Check sheet for the drawn part. Datum: minimum x, y, z corner. Units: mm. Round coordinates to 2 decimals unless told otherwise and drop trailing zeros. Order: outer loops, then holes, each group sorted by start corner. A loop starts at its lowest first (then second) coordinate and runs counter-clockwise, first axis right, second up.
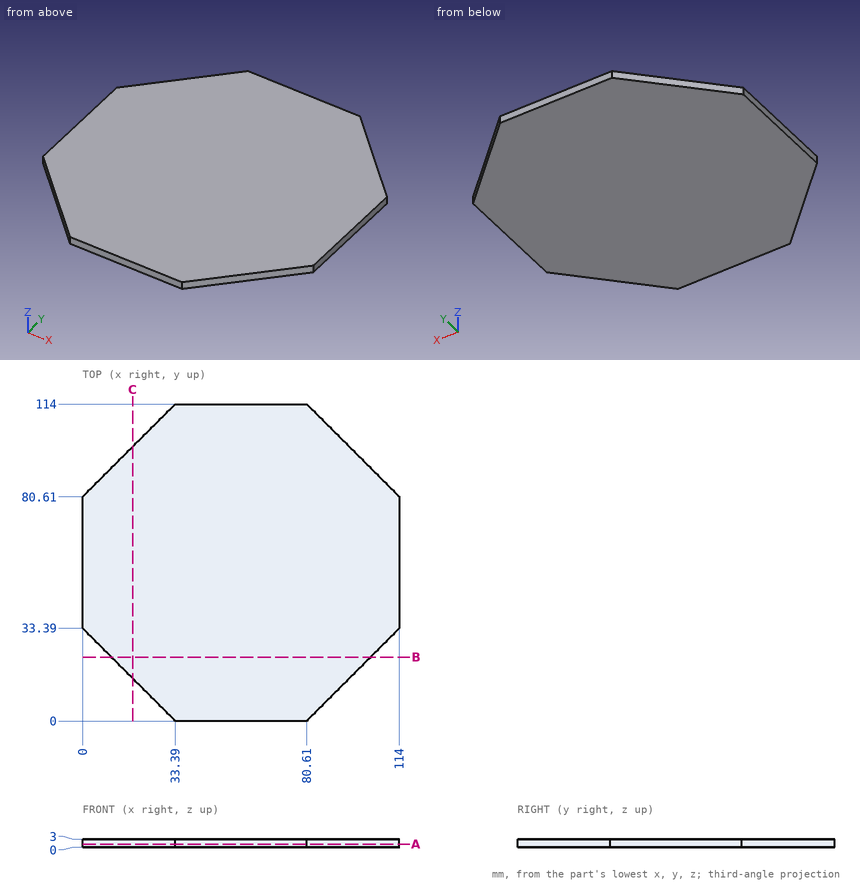
(1) Sectioned sample at A-A, the plane z = 1.2. Record the cut outline in (x, y), and give its area (3 significant figures).
Returned:
outline: (0, 33.39) - (33.39, 0) - (80.61, 0) - (114, 33.39) - (114, 80.61) - (80.61, 114) - (33.39, 114) - (0, 80.61) - close
area: 10,800 mm2
(2) Material ranges on line 1 (X direction, y = 11, z = 1.05); line 2 (X direction, y = 27, z = 2.35); line 3 (Y direction, x = 12, z = 0.4), recorded low to high.
Returned:
line 1: x = 22.39 to 91.61
line 2: x = 6.39 to 107.61
line 3: y = 21.39 to 92.61
(3) Sectioned sample at B-B, the plane y = 23. Record the cut outline in (x, z), and give its area (3 significant figures).
Returned:
outline: (10.39, 0) - (103.61, 0) - (103.61, 3) - (10.39, 3) - close
area: 280 mm2
(4) Sectioned sample at C-C, the plane x = 18. Record the cut outline in (y, z), and give its area (3 significant figures).
Returned:
outline: (15.39, 0) - (98.61, 0) - (98.61, 3) - (15.39, 3) - close
area: 250 mm2
